CAD build for the part. Positions are in the model's coordinates, mm. A direction names the side the tool comes from. Coordinates: 2 decimals unless noted, no trailing zeros. Write each loop counter-clockwise with the first axis right and the second up, starting at its lowest first coordinate (ties: lowest second). Pieces come first, ordered by that corner, then holes. Notation, with made-up numbers: (10, 88) - (69, 88) arc R21 cw to (69, 112) - close; hole circle Ø1 at (36, -27). An arc over 180 degrees is marked (long way). Answer in a Markdown table with one row per item. Add a question column.
Q1. Pin check, flat tips, straight feed: pin 1 (2 mm diameter, centred on x = 6.5, y = -0.5, fed in from -Z); pin 2 (0.6 mm diameter, centred on x = 14.5, y = 1, fed in from -Z); pin 3 (1.5 mm diameter, centred on x = 5, y = 2.5, fed in from +Z). Stop position of each tip, or through.
Q2. Drill centre lines: line 1 along X through (y, z) = (-1.25, 5); line 2 along X through (y, z) = (-2, 15); line 3 along X through (y, z) = (1, 13.5). Where is each one in solid material? Low to high. Write a range as from..to.
Q3. Band-saw the part on B-B (x = 22). List the corners of the cut face in (y, z).
Q4. 3-axis set-ups, long thin cutter, end or side, ignore diameter. For faces 4 (the flat face through (33, 0, 16.495)), 5 (the cylindrical face through (-6.23, -0.06, 11.97)), 6 (the flat face through (-31.509, -0.056, 9.573)), 7 (the flat face through (-3, 0, 6.25)), 8 (the flat face through (26, 0, 0)): which of +Z, -Z, +X, -X, +Y, -Y reach the whole face in a straight line?
Q5. Band-saw the part on C-C (x = -27). List the corners of the cut face in (y, z), and give its area (3 significant figures).
Q6. Two-plate mould, pull along Z, no slides. Class faces 1 (the flat face through (-1, 4, 7)), 2 (the cylindrical face through (-16.49, -0.06, 11.05)), 3 (the flat face through (-33, 0, 16.495)): +Z half, -Z half, draft (parallel to the pull), parting line (faces both ways), or undercut.
Q7. Band-saw the part on A-A (z = 3.5). List the corners of the cut face in (x, y).
```python
from build123d import *

# Parameters (mm, degrees)
F2_DEPTH = 4
F3_R     = 1
F4_R     = 0.25


# Not quite as in the source:
# - a feature names something its author has since deleted; it is built from what else it names


with BuildPart() as f2:
    # F1 (on Front) → F2 (new body, symmetric)
    with BuildSketch(Plane.XZ):
        with BuildLine():
            Line((-37.5, 16.4951905284), (-37.5, 0))
            Line((-37.5, 0), (-4.4515441619, 0))
            Line((-4.4515441619, 0), (-4.4515441619, 6.25))
            Line((-4.4515441619, 6.25), (-2.4515441619, 6.25))
            Line((-2.4515441619, 6.25), (-2.4515441619, 2.25))
            Line((-2.4515441619, 2.25), (13.5484558381, 2.25))
            Line((13.5484558381, 2.25), (13.5484558381, 6.25))
            Line((13.5484558381, 6.25), (15.5484558381, 6.25))
            Line((15.5484558381, 6.25), (15.5484558381, 0))
            Line((15.5484558381, 0), (37.5, 0))
            Line((37.5, 0), (37.5, 16.4951905284))
            Line((37.5, 16.4951905284), (29.0959722333, 16.4951905284))
            Line((29.0959722333, 16.4951905284), (31.6940484447, 14.9951905284))
            Line((31.6940484447, 14.9951905284), (31.9440484447, 15.4282032303))
            Line((31.9440484447, 15.4282032303), (34.542124656, 13.9282032303))
            Line((34.542124656, 13.9282032303), (30.542124656, 7))
            ThreePointArc((30.542124656, 7), (26.5409294992, 7.164032547), (22.7969341276, 8.5849364905))
            Line((22.7969341276, 8.5849364905), (9.0959722333, 16.4951905284))
            Line((9.0959722333, 16.4951905284), (8.0959722333, 16.4951905284))
            Line((8.0959722333, 16.4951905284), (9.5959722333, 13.897114317))
            Line((9.5959722333, 13.897114317), (10.0289849352, 14.147114317))
            Line((10.0289849352, 14.147114317), (11.5289849352, 11.5490381057))
            Line((11.5289849352, 11.5490381057), (4.6007817049, 7.5490381057))
            ThreePointArc((4.6007817049, 7.5490381057), (1.2176613272, 9.6916920368), (-1.3142818045, 12.7942286341))
            Line((-1.3142818045, 12.7942286341), (-3.4510331505, 16.4951905284))
            Line((-3.4510331505, 16.4951905284), (-4.4510331505, 16.4951905284))
            Line((-4.4510331505, 16.4951905284), (-4.756308124, 15.3558888168))
            ThreePointArc((-4.756308124, 15.3558888168), (-6.3989818261, 11.7037534869), (-9.112265528, 8.7584927324))
            Line((-9.112265528, 8.7584927324), (-16.8396721383, 10.8290450932))
            Line((-16.8396721383, 10.8290450932), (-16.063215003, 13.7268225721))
            Line((-16.063215003, 13.7268225721), (-15.5802520899, 13.5974130495))
            Line((-15.5802520899, 13.5974130495), (-14.8037949546, 16.4951905284))
            Line((-14.8037949546, 16.4951905284), (-15.8037949546, 16.4951905284))
            Line((-15.8037949546, 16.4951905284), (-21.8142025947, 10.4847828883))
            ThreePointArc((-21.8142025947, 10.4847828883), (-25.0628674157, 8.1432777656), (-28.8852704065, 6.9492489824))
            Line((-28.8852704065, 6.9492489824), (-34.542124656, 12.6061032319))
            Line((-34.542124656, 12.6061032319), (-32.4208043125, 14.7274235754))
            Line((-32.4208043125, 14.7274235754), (-32.0672509219, 14.3738701848))
            Line((-32.0672509219, 14.3738701848), (-29.9459305783, 16.4951905284))
            Line((-29.9459305783, 16.4951905284), (-37.5, 16.4951905284))
        make_face()
    extrude(amount=F2_DEPTH, both=True)

    # F3
    f3_edges = [f2.edges().sort_by_distance(p)[0] for p in [
        (-37.5, 0, 0),
        (37.5, 0, 0),
        (37.5, 0, 16.495191),
        (9.095972, 0, 16.495191),
        (30.542125, 0, 7),
        (4.600782, 0, 7.549038),
        (34.542125, 0, 13.928203),
        (-9.112266, 0, 8.758493),
        (-28.88527, 0, 6.949249),
        (-3.451033, 0, 16.495191),
        (-1.314282, 0, 12.794229),
        (-15.803795, 0, 16.495191),
        (-37.5, 0, 16.495191),
        (11.528985, 0, 11.549038),
        (-16.839672, 0, 10.829045),
        (-34.542125, 0, 12.606103),
    ]]
    fillet(f3_edges, radius=F3_R)

    # F4
    f4_edges = [f2.edges().sort_by_distance(p)[0] for p in [
        (29.095972, 0, 16.495191),
        (-4.451033, 0, 16.495191),
        (-14.803795, 0, 16.495191),
        (-29.945931, 0, 16.495191),
        (31.694048, 0, 14.995191),
        (-15.580252, 0, 13.597413),
        (-32.067251, 0, 14.37387),
        (9.595972, 0, 13.897114),
        (8.095972, 0, 16.495191),
    ]]
    fillet(f4_edges, radius=F4_R)


solid = f2.part
```
Checked values:
| question | item | result |
|---|---|---|
| 1 | pin 1 | stops at z = 2.25 |
| 1 | pin 2 | stops at z = 6.25 |
| 1 | pin 3 | stops at z = 8.21 |
| 2 | line 1 | x = -37.5..-4.45, -2.45..13.55, 15.55..37.5 |
| 2 | line 2 | x = -37.5..-31.44, -17.3..-15.2, -4.86..-2.59, 8.96..11.69, 32.69..37.5 |
| 2 | line 3 | x = -37.5..-33.65, -18.8..-16.12, -5.41..-1.72, 10.4..14.28, 34.17..37.5 |
| 3 | outline | (-4, 0) - (4, 0) - (4, 9.05) - (-4, 9.05) - close |
| 4 | face 4 | +Z, +X, -X, +Y, -Y |
| 4 | face 5 | +Z, +Y, -Y |
| 4 | face 6 | +Y, -Y |
| 4 | face 7 | -Z, +Y, -Y |
| 4 | face 8 | -Z, +X, -X, +Y, -Y |
| 5 | outline | (-4, 0) - (4, 0) - (4, 7.37) - (-4, 7.37) - close |
| 5 | area | 59.0 mm² |
| 6 | face 1 | draft |
| 6 | face 2 | undercut |
| 6 | face 3 | +Z half |
| 7 | outline | (-37.5, -4) - (-4.45, -4) - (-4.45, 4) - (-37.5, 4) - close; (-2.45, -4) - (13.55, -4) - (13.55, 4) - (-2.45, 4) - close; (15.55, -4) - (37.5, -4) - (37.5, 4) - (15.55, 4) - close |
